from build123d import *

# Parameters (mm, degrees)
F1_DEPTH = 5


with BuildPart() as f1:
    # F0 (on Top) → F1 (new body)
    with BuildSketch(Plane.XY):
        with BuildLine():
            ThreePointArc((-2.674113, -54.37004), (-0.770343, -53.970695), (0.836963, -52.875074))
            Line((0.836963, -52.875074), (88.193572, 36.010466))
            ThreePointArc((88.193572, 36.010466), (88.611566, 38.185732), (86.767144, 39.412358))
            Line((86.767144, 39.412358), (83.100055, 39.412358))
            ThreePointArc((83.100055, 39.412358), (79.100055, 43.412358), (83.100055, 47.412358))
            Line((83.100055, 47.412358), (86.767144, 47.454403))
            ThreePointArc((86.767144, 47.454403), (88.767144, 49.454403), (86.767144, 51.454403))
            Line((86.767144, 51.454403), (71.387003, 51.454403))
            Line((71.387003, 51.454403), (24.701984, 6.277601))
            ThreePointArc((24.701984, 6.277601), (23.703334, 5.528153), (22.550135, 5.049502))
            Line((22.550135, 5.049502), (-68.458309, -19.965363))
            ThreePointArc((-68.458309, -19.965363), (-69.412453, -20.609364), (-69.781248, -21.699831))
            Line((-69.781248, -21.699831), (-69.786822, -30.330341))
            ThreePointArc((-69.786822, -30.330341), (-69.201493, -31.74539), (-67.786822, -32.331633))
            Line((-67.786822, -32.331633), (-63.788114, -32.331633))
            ThreePointArc((-63.788114, -32.331633), (-62.373901, -31.745846), (-61.788114, -30.331633))
            Line((-61.788114, -30.331633), (-61.788114, -27.331633))
            Line((-61.788114, -27.331633), (-21.788114, -27.331633))
            Line((-21.788114, -27.331633), (-21.788114, -46.331633))
            Line((-21.788114, -46.331633), (-29.788114, -46.331633))
            ThreePointArc((-29.788114, -46.331633), (-31.202328, -46.917419), (-31.788114, -48.331633))
            Line((-31.788114, -48.331633), (-31.788114, -52.668167))
            ThreePointArc((-31.788114, -52.668167), (-31.194529, -54.090137), (-29.766116, -54.668046))
            Line((-29.766116, -54.668046), (-2.674113, -54.37004))
        make_face()
        with BuildLine():
            Line((-13.958797, -35.468011), (-7.226438, -45.566549))
            ThreePointArc((-7.226438, -45.566549), (-7.138692, -47.640851), (-8.938748, -48.675368))
            Line((-8.938748, -48.675368), (-15.671107, -48.513038))
            ThreePointArc((-15.671107, -48.513038), (-17.054054, -47.910684), (-17.622897, -46.513619))
            Line((-17.622897, -46.513619), (-17.622897, -36.577411))
            ThreePointArc((-17.622897, -36.577411), (-16.202466, -34.663227), (-13.958797, -35.468011))
        make_face(mode=Mode.SUBTRACT)
        with BuildLine():
            ThreePointArc((-10.975061, -34.104397), (-11.085903, -32.045596), (-9.319116, -30.982859))
            Line((-9.319116, -30.982859), (10.997215, -30.982859))
            ThreePointArc((10.997215, -30.982859), (12.855047, -32.242277), (12.373093, -34.434397))
            Line((12.373093, -34.434397), (0, -46.162553))
            ThreePointArc((0, -46.162553), (-1.59229, -46.699272), (-3.031822, -45.832553))
            Line((-3.031822, -45.832553), (-10.975061, -34.104397))
        make_face(mode=Mode.SUBTRACT)
        with BuildLine():
            Line((-10.519725, -11.797756), (-17.826055, -22.051859))
            ThreePointArc((-17.826055, -22.051859), (-18.5489, -22.674313), (-19.477843, -22.891148))
            Line((-19.477843, -22.891148), (-45.430275, -22.593101))
            ThreePointArc((-45.430275, -22.593101), (-47.387827, -20.871703), (-45.980863, -18.677238))
            Line((-45.980863, -18.677238), (-12.722101, -8.721183))
            ThreePointArc((-12.722101, -8.721183), (-10.522285, -9.473013), (-10.519725, -11.797756))
        make_face(mode=Mode.SUBTRACT)
        with BuildLine():
            Line((12.215566, -27.616652), (-12.687871, -26.858329))
            ThreePointArc((-12.687871, -26.858329), (-14.436563, -25.711004), (-14.206369, -23.632232))
            Line((-14.206369, -23.632232), (-3.058227, -9.282833))
            ThreePointArc((-3.058227, -9.282833), (-1.556912, -8.511381), (0, -9.163386))
            Line((0, -9.163386), (13.755295, -24.271108))
            ThreePointArc((13.755295, -24.271108), (14.093259, -26.453739), (12.215566, -27.616652))
        make_face(mode=Mode.SUBTRACT)
        with BuildLine():
            Line((19.271857, -2.765768), (19.271857, -20.532251))
            ThreePointArc((19.271857, -20.532251), (17.953823, -22.41239), (15.736935, -21.814441))
            Line((15.736935, -21.814441), (4.052052, -7.826359))
            ThreePointArc((4.052052, -7.826359), (3.665453, -5.989415), (4.97163, -4.641184))
            Line((4.97163, -4.641184), (16.656512, -0.862783))
            ThreePointArc((16.656512, -0.862783), (18.448571, -1.148565), (19.271857, -2.765768))
        make_face(mode=Mode.SUBTRACT)
        with BuildLine():
            Line((25.136737, 1.298854), (43.714296, 1.298854))
            ThreePointArc((43.714296, 1.298854), (45.559407, 0.070584), (45.138224, -2.105579))
            Line((45.138224, -2.105579), (26.389468, -21.114586))
            ThreePointArc((26.389468, -21.114586), (24.315692, -21.538242), (23.136737, -19.780375))
            Line((23.136737, -19.780375), (23.136737, -0.701146))
            ThreePointArc((23.136737, -0.701146), (23.722523, 0.713067), (25.136737, 1.298854))
        make_face(mode=Mode.SUBTRACT)
        with BuildLine():
            ThreePointArc((53.998229, 7.187327), (53.412442, 5.773113), (51.998229, 5.187327))
            Line((51.998229, 5.187327), (33.807475, 5.187327))
            ThreePointArc((33.807475, 5.187327), (31.9603, 6.42055), (32.391104, 8.59938))
            Line((32.391104, 8.59938), (50.581858, 26.845761))
            ThreePointArc((50.581858, 26.845761), (52.762185, 27.282051), (53.998229, 25.433708))
            Line((53.998229, 25.433708), (53.998229, 7.187327))
        make_face(mode=Mode.SUBTRACT)
        with BuildLine():
            Line((59.283667, 33.462164), (76.083784, 33.462164))
            ThreePointArc((76.083784, 33.462164), (77.930966, 32.228923), (77.500126, 30.050083))
            Line((77.500126, 30.050083), (60.700009, 13.199277))
            ThreePointArc((60.700009, 13.199277), (58.519692, 12.763024), (57.283667, 14.611359))
            Line((57.283667, 14.611359), (57.283667, 31.462164))
            ThreePointArc((57.283667, 31.462164), (57.869453, 32.876378), (59.283667, 33.462164))
        make_face(mode=Mode.SUBTRACT)
        with BuildLine():
            Line((76.341538, 45.880931), (76.341538, 38.404973))
            ThreePointArc((76.341538, 38.404973), (75.736125, 36.971401), (74.28641, 36.405733))
            Line((74.28641, 36.405733), (67.249003, 36.599787))
            ThreePointArc((67.249003, 36.599787), (65.439989, 37.874478), (65.913325, 40.036266))
            Line((65.913325, 40.036266), (73.289812, 47.174446))
            ThreePointArc((73.289812, 47.174446), (75.243995, 47.538204), (76.341538, 45.880931))
        make_face(mode=Mode.SUBTRACT)
    extrude(amount=F1_DEPTH)


solid = f1.part
Work out the finished part from the listing and answer in its coordinate system (mm). A direction names the side the tool comes from. Coordinates: 2 decimals unless noted, no trailing zeros. Loops run counter-clockwise (first coordinate to the right, second up) from the corner with the lowest first, then second, coordinate; pieces in that order, holes last. Notation, with made-up numbers: M 56.5,4.5 L 93.5,4.5 A22 ccw 93.5,13.5 Z; hole C -22,-11 d4. An arc over 180 degrees is marked long. Answer in a Markdown table with one row per item. Add a question column.
1. The mould has two halves that part along Y. Classify faces 1 (the flat face through (-66, -32.332, 2)), 2 (the flat face through (-42, -27.332, 2)), 3 (the flat face through (-61.788, -29, 2)): pulls with the +Y half, pulls with the -Y half, needs draft (parallel to the pull), parting line crosses it, or undercut.
2. Find section C-C, the plane z = 1. State how many separate pieces and enclosed holes the cut face has, then the cut area to 3 significant figures.
3. Find section B-B, the plane x = -43. Write down the section's boundary in (y, z).
4. Consider L1, parallel to Y at x = -13, z = 2.55; L2, parallel to X at y = -37.5, z = 2.1; L3, parallel to Y at x = 9.5, z = 0.8. Determine where each line is inside the solid, lowest interval first.
5. Find section D-D, the plane x = 63. Write down the section's boundary in (y, z).
6. Find section A-A, the plane y = -14.5. Write down the section's boundary in (x, z), then the cut area to 3 significant figures.
7. Flat-ended cylindrical pins translate along their axes: P1, Ø1.5, axis at x = -40, z = 2, coming from the -Y side; P2, Ø2.5, axis at y = -39, z = 3.5, coming from the -X side; P3, Ø2.5, axis at x = 40.5, z = 3, coming from the +Y side. Find the tip coordinate at first contact, or state that the pin passes through.
8. A tool of negligible diameter and unlimited length cuts with its end or side. For faces 4 (the flat face through (15, -1, 5)), 5 (the flat face through (10.73, -2.78, 2.46)), from which of +Z, -Z, +X, -X, +Y, -Y can it reach the whole face along a straight path? Write none if from no direction.
Reported:
| question | item | result |
|---|---|---|
| 1 | face 1 | pulls with the -Y half |
| 1 | face 2 | undercut |
| 1 | face 3 | needs draft |
| 2 | separate pieces | 1 |
| 2 | enclosed holes | 9 |
| 2 | area | 2,710 mm^2 |
| 3 | outline | M -27.33,0 L -22.62,0 L -22.62,5 L -27.33,5 Z; M -17.78,0 L -12.97,0 L -12.97,5 L -17.78,5 Z |
| 4 | L1 | y = -54.48 to -48.58, -36.91 to -26.82, -22.08 to -15.28, -8.8 to -4.72 |
| 4 | L2 | x = -21.79 to -17.62, -12.6 to -8.68, 9.14 to 15.95 |
| 4 | L3 | y = -44.06 to -37.16, -30.98 to -27.53, -19.6 to -14.35, -3.18 to 1.46 |
| 5 | outline | M 10.38,0 L 15.51,0 L 15.51,5 L 10.38,5 Z; M 33.46,0 L 43.34,0 L 43.34,5 L 33.46,5 Z |
| 6 | outline | M -48.57,0 L -32.03,0 L -32.03,5 L -48.57,5 Z; M -12.45,0 L -7.11,0 L -7.11,5 L -12.45,5 Z; M 4.86,0 L 9.63,0 L 9.63,5 L 4.86,5 Z; M 19.27,0 L 23.14,0 L 23.14,5 L 19.27,5 Z; M 32.91,0 L 38.55,0 L 38.55,5 L 32.91,5 Z |
| 6 | area | 181 mm^2 |
| 7 | P1 | stops at y = -27.33 |
| 7 | P2 | stops at x = -21.79 |
| 7 | P3 | stops at y = 22.77 |
| 8 | face 4 | +Z, +X, -X, +Y, -Y |
| 8 | face 5 | +Z, -Z |
